The listing builds one solid part. Answer for the finished solid, in the listing's coordinates (mm). Give positions to 0.01 mm unless a question says otherwise; leave off trailing zeros. Write each loop counter-clockwise with the first axis right and the second up, starting at its lowest first coordinate (ties: lowest second). Pieces come first, ordered by that corner, then holes. Notation, with made-up numbers: (-19.75, 13) - (35.25, 13) arc R6 ccw to (35.25, 21) - close; hole circle Ø11 at (39, -26). An arc over 180 degrees is marked (long way). Write each question's results on one line, items separated by ' | '. Start each with the question number.
Q1. Section A-A (z = 0) is taken. Determine the outline of the cut face in (x, y).
Q2. Flat-ended cylindrical pins translate along their axes: pin 1 Ø2 at (y, z) = (2.5, -91) entering from +X; pin 2 Ø2 at (x, y) = (23, 2) entering from +Z. Find the tip coordinate at first contact, or state that the pin passes through.
Q3. Section B-B (y = 0.95) is taken. State how many separate pieces and enclosed holes the cut face has, plus the area to 3 significant figures.
Q4. Find the intervals of material crossed by probe 1 along X at (y, z) = (1, -36.5); probe 2 along Z at (x, y) = (84.5, 2.55); probe 3 along Z at (x, y) = (79.5, 0.35), in increasing order.
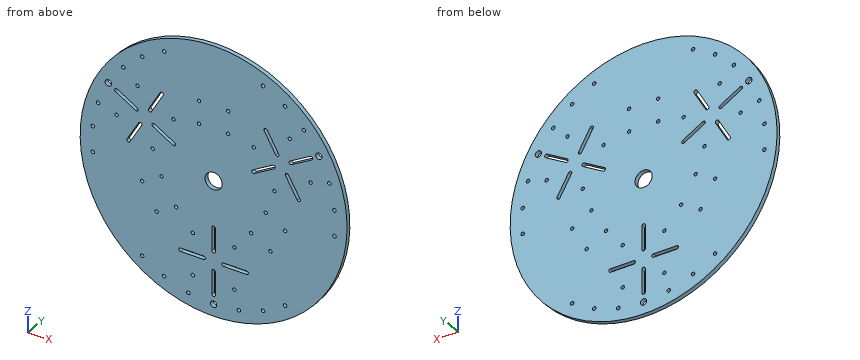
```python
from build123d import *

# Parameters (mm, degrees)
SKETCH1_R           = 125
SKETCH1_R_2         = 8
SKETCH1_R_3         = 2.95
SKETCH1_R_4         = 1.675
SKETCH1_R_5         = 1.6
BOSS_EXTRUDE2_DEPTH = 4


with BuildPart() as part:
    # Sketch1 → Boss-Extrude2 (new body)
    with BuildSketch(Plane(origin=(0, 0, 0), x_dir=(1, 0, 0), z_dir=(0, 1, 0))):
        with Locations(Location((0, 0, 0), (0, 0, 270))):
            Circle(SKETCH1_R)
        with Locations(Location((0, 0, 0), (0, 0, 270))):
            Circle(SKETCH1_R_2, mode=Mode.SUBTRACT)
        with Locations(Location((0, 113.85, 0), (0, 0, 270))):
            Circle(SKETCH1_R_3, mode=Mode.SUBTRACT)
        with Locations(Location((98.596992221, -56.925, 0), (0, 0, 270))):
            Circle(SKETCH1_R_3, mode=Mode.SUBTRACT)
        with Locations(Location((-98.596992221, -56.925, 0), (0, 0, 270))):
            Circle(SKETCH1_R_3, mode=Mode.SUBTRACT)
        with Locations(Location((23.670746, 111.362104344, 0), (0, 0, 270))):
            Circle(SKETCH1_R_4, mode=Mode.SUBTRACT)
        with Locations(Location((46.306966814, 104.007150353, 0), (0, 0, 270))):
            Circle(SKETCH1_R_4, mode=Mode.SUBTRACT)
        with Locations(Location((66.919350973, 92.10658481, 0), (0, 0, 270))):
            Circle(SKETCH1_R_4, mode=Mode.SUBTRACT)
        with Locations(Location((113.226317788, 11.900565543, 0), (0, 0, 270))):
            Circle(SKETCH1_R_4, mode=Mode.SUBTRACT)
        with Locations(Location((113.226317788, -11.900565543, 0), (0, 0, 270))):
            Circle(SKETCH1_R_4, mode=Mode.SUBTRACT)
        with Locations(Location((108.27778438, -35.18158481, 0), (0, 0, 270))):
            Circle(SKETCH1_R_4, mode=Mode.SUBTRACT)
        with Locations(Location((84.607038381, -76.180519534, 0), (0, 0, 270))):
            Circle(SKETCH1_R_4, mode=Mode.SUBTRACT)
        with Locations(Location((66.919350974, -92.10658481, 0), (0, 0, 270))):
            Circle(SKETCH1_R_4, mode=Mode.SUBTRACT)
        with Locations(Location((46.306966814, -104.007150353, 0), (0, 0, 270))):
            Circle(SKETCH1_R_4, mode=Mode.SUBTRACT)
        with Locations(Location((-46.306966814, -104.007150353, 0), (0, 0, 270))):
            Circle(SKETCH1_R_4, mode=Mode.SUBTRACT)
        with Locations(Location((-66.919350973, -92.10658481, 0), (0, 0, 270))):
            Circle(SKETCH1_R_4, mode=Mode.SUBTRACT)
        with Locations(Location((-84.607038381, -76.180519534, 0), (0, 0, 270))):
            Circle(SKETCH1_R_4, mode=Mode.SUBTRACT)
        with Locations(Location((-108.27778438, -35.18158481, 0), (0, 0, 270))):
            Circle(SKETCH1_R_4, mode=Mode.SUBTRACT)
        with Locations(Location((-113.226317788, -11.900565543, 0), (0, 0, 270))):
            Circle(SKETCH1_R_4, mode=Mode.SUBTRACT)
        with Locations(Location((-113.226317788, 11.900565543, 0), (0, 0, 270))):
            Circle(SKETCH1_R_4, mode=Mode.SUBTRACT)
        with Locations(Location((-66.919350973, 92.10658481, 0), (0, 0, 270))):
            Circle(SKETCH1_R_4, mode=Mode.SUBTRACT)
        with Locations(Location((-46.306966814, 104.007150353, 0), (0, 0, 270))):
            Circle(SKETCH1_R_4, mode=Mode.SUBTRACT)
        with Locations(Location((-23.670746, 111.362104344, 0), (0, 0, 270))):
            Circle(SKETCH1_R_4, mode=Mode.SUBTRACT)
        with Locations(Location((-90.831628429, -29.925004626, 0), (0, 0, 270))):
            Circle(SKETCH1_R_5, mode=Mode.SUBTRACT)
        with Locations(Location((-57.056637682, -10.425004626, 0), (0, 0, 270))):
            Circle(SKETCH1_R_5, mode=Mode.SUBTRACT)
        with Locations(Location((-37.556637682, -44.199995374, 0), (0, 0, 270))):
            Circle(SKETCH1_R_5, mode=Mode.SUBTRACT)
        with Locations(Location((-71.331628429, -63.699995374, 0), (0, 0, 270))):
            Circle(SKETCH1_R_5, mode=Mode.SUBTRACT)
        with Locations(Location((19.5, 93.625, 0), (0, 0, 270))):
            Circle(SKETCH1_R_5, mode=Mode.SUBTRACT)
        with Locations(Location((19.5, 54.625, 0), (0, 0, 270))):
            Circle(SKETCH1_R_5, mode=Mode.SUBTRACT)
        with Locations(Location((-19.5, 54.625, 0), (0, 0, 270))):
            Circle(SKETCH1_R_5, mode=Mode.SUBTRACT)
        with Locations(Location((-19.5, 93.625, 0), (0, 0, 270))):
            Circle(SKETCH1_R_5, mode=Mode.SUBTRACT)
        with Locations(Location((71.331628429, -63.699995374, 0), (0, 0, 270))):
            Circle(SKETCH1_R_5, mode=Mode.SUBTRACT)
        with Locations(Location((37.556637682, -44.199995374, 0), (0, 0, 270))):
            Circle(SKETCH1_R_5, mode=Mode.SUBTRACT)
        with Locations(Location((57.056637682, -10.425004626, 0), (0, 0, 270))):
            Circle(SKETCH1_R_5, mode=Mode.SUBTRACT)
        with Locations(Location((90.831628429, -29.925004626, 0), (0, 0, 270))):
            Circle(SKETCH1_R_5, mode=Mode.SUBTRACT)
        with Locations(Location((-13.625, -48.465, 0), (0, 0, 270))):
            Circle(SKETCH1_R_5, mode=Mode.SUBTRACT)
        with Locations(Location((13.625, -48.465, 0), (0, 0, 270))):
            Circle(SKETCH1_R_5, mode=Mode.SUBTRACT)
        with Locations(Location((13.625, -69.465, 0), (0, 0, 270))):
            Circle(SKETCH1_R_5, mode=Mode.SUBTRACT)
        with Locations(Location((-13.625, -69.465, 0), (0, 0, 270))):
            Circle(SKETCH1_R_5, mode=Mode.SUBTRACT)
        with Locations(Location((-35.159421194, 36.032096127, 0), (0, 0, 270))):
            Circle(SKETCH1_R_5, mode=Mode.SUBTRACT)
        with Locations(Location((-48.784421194, 12.432903873, 0), (0, 0, 270))):
            Circle(SKETCH1_R_5, mode=Mode.SUBTRACT)
        with Locations(Location((-66.970954674, 22.932903873, 0), (0, 0, 270))):
            Circle(SKETCH1_R_5, mode=Mode.SUBTRACT)
        with Locations(Location((-53.345954674, 46.532096127, 0), (0, 0, 270))):
            Circle(SKETCH1_R_5, mode=Mode.SUBTRACT)
        with Locations(Location((48.784421194, 12.432903873, 0), (0, 0, 270))):
            Circle(SKETCH1_R_5, mode=Mode.SUBTRACT)
        with Locations(Location((35.159421194, 36.032096127, 0), (0, 0, 270))):
            Circle(SKETCH1_R_5, mode=Mode.SUBTRACT)
        with Locations(Location((53.345954674, 46.532096127, 0), (0, 0, 270))):
            Circle(SKETCH1_R_5, mode=Mode.SUBTRACT)
        with Locations(Location((66.970954674, 22.932903873, 0), (0, 0, 270))):
            Circle(SKETCH1_R_5, mode=Mode.SUBTRACT)
        with BuildLine():
            Line((-71.383217405, -43.060640646), (-90.262571208, -53.960640646))
            ThreePointArc((-90.262571208, -53.960640646), (-92.448211854, -53.375), (-91.862571208, -51.189359354))
            Line((-91.862571208, -51.189359354), (-72.983217405, -40.289359354))
            ThreePointArc((-72.983217405, -40.289359354), (-70.797576759, -40.875), (-71.383217405, -43.060640646))
        make_face(mode=Mode.SUBTRACT)
        with BuildLine():
            Line((-36.525694903, -22.935640646), (-55.405048706, -33.835640646))
            ThreePointArc((-55.405048706, -33.835640646), (-57.590689352, -33.25), (-57.005048706, -31.064359354))
            Line((-57.005048706, -31.064359354), (-38.125694903, -20.164359354))
            ThreePointArc((-38.125694903, -20.164359354), (-35.940054257, -20.75), (-36.525694903, -22.935640646))
        make_face(mode=Mode.SUBTRACT)
        with BuildLine():
            Line((-70.192273702, -29.87341565), (-81.092273702, -10.994061848))
            ThreePointArc((-81.092273702, -10.994061848), (-80.506633056, -8.808421202), (-78.320992409, -9.394061848))
            Line((-78.320992409, -9.394061848), (-67.420992409, -28.27341565))
            ThreePointArc((-67.420992409, -28.27341565), (-68.006633056, -30.459056296), (-70.192273702, -29.87341565))
        make_face(mode=Mode.SUBTRACT)
        with BuildLine():
            Line((-58.195992409, -44.25158435), (-47.295992409, -63.130938152))
            ThreePointArc((-47.295992409, -63.130938152), (-47.881633056, -65.316578798), (-50.067273702, -64.730938152))
            Line((-50.067273702, -64.730938152), (-60.967273702, -45.85158435))
            ThreePointArc((-60.967273702, -45.85158435), (-60.381633056, -43.665943704), (-58.195992409, -44.25158435))
        make_face(mode=Mode.SUBTRACT)
        with BuildLine():
            Line((-1.6, 83.35), (-1.6, 105.15))
            ThreePointArc((-1.6, 105.15), (0, 106.75), (1.6, 105.15))
            Line((1.6, 105.15), (1.6, 83.35))
            ThreePointArc((1.6, 83.35), (0, 81.75), (-1.6, 83.35))
        make_face(mode=Mode.SUBTRACT)
        with BuildLine():
            Line((-1.6, 43.1), (-1.6, 64.9))
            ThreePointArc((-1.6, 64.9), (0, 66.5), (1.6, 64.9))
            Line((1.6, 64.9), (1.6, 43.1))
            ThreePointArc((1.6, 43.1), (0, 41.5), (-1.6, 43.1))
        make_face(mode=Mode.SUBTRACT)
        with BuildLine():
            Line((9.225, 75.725), (31.025, 75.725))
            ThreePointArc((31.025, 75.725), (32.625, 74.125), (31.025, 72.525))
            Line((31.025, 72.525), (9.225, 72.525))
            ThreePointArc((9.225, 72.525), (7.625, 74.125), (9.225, 75.725))
        make_face(mode=Mode.SUBTRACT)
        with BuildLine():
            Line((-9.225, 72.525), (-31.025, 72.525))
            ThreePointArc((-31.025, 72.525), (-32.625, 74.125), (-31.025, 75.725))
            Line((-31.025, 75.725), (-9.225, 75.725))
            ThreePointArc((-9.225, 75.725), (-7.625, 74.125), (-9.225, 72.525))
        make_face(mode=Mode.SUBTRACT)
        with BuildLine():
            Line((72.983217405, -40.289359354), (91.862571208, -51.189359354))
            ThreePointArc((91.862571208, -51.189359354), (92.448211854, -53.375), (90.262571208, -53.960640646))
            Line((90.262571208, -53.960640646), (71.383217405, -43.060640646))
            ThreePointArc((71.383217405, -43.060640646), (70.797576759, -40.875), (72.983217405, -40.289359354))
        make_face(mode=Mode.SUBTRACT)
        with BuildLine():
            Line((38.125694903, -20.164359354), (57.005048706, -31.064359354))
            ThreePointArc((57.005048706, -31.064359354), (57.590689352, -33.25), (55.405048706, -33.835640646))
            Line((55.405048706, -33.835640646), (36.525694903, -22.935640646))
            ThreePointArc((36.525694903, -22.935640646), (35.940054257, -20.75), (38.125694903, -20.164359354))
        make_face(mode=Mode.SUBTRACT)
        with BuildLine():
            Line((60.967273702, -45.85158435), (50.067273702, -64.730938152))
            ThreePointArc((50.067273702, -64.730938152), (47.881633056, -65.316578798), (47.295992409, -63.130938152))
            Line((47.295992409, -63.130938152), (58.195992409, -44.25158435))
            ThreePointArc((58.195992409, -44.25158435), (60.381633056, -43.665943704), (60.967273702, -45.85158435))
        make_face(mode=Mode.SUBTRACT)
        with BuildLine():
            Line((67.420992409, -28.27341565), (78.320992409, -9.394061848))
            ThreePointArc((78.320992409, -9.394061848), (80.506633056, -8.808421202), (81.092273702, -10.994061848))
            Line((81.092273702, -10.994061848), (70.192273702, -29.87341565))
            ThreePointArc((70.192273702, -29.87341565), (68.006633056, -30.459056296), (67.420992409, -28.27341565))
        make_face(mode=Mode.SUBTRACT)
    extrude(amount=BOSS_EXTRUDE2_DEPTH)


solid = part.part
```
Answers below:
1) outline: (-125, 0) - (-8, 0) - (-8, 4) - (-125, 4) - close; (8, 0) - (125, 0) - (125, 4) - (8, 4) - close
2) pin 1: stops at x = 86.75 | pin 2: stops at z = 123.05
3) separate pieces: 1 | enclosed holes: 58 | area: 47,500 mm2
4) probe 1: x = -119.55 to -36.69, -33.63 to 33.63, 36.69 to 119.55 | probe 2: z = -92.11 to 46.94, 50.63 to 74.51, 77.85 to 92.11 | probe 3: z = -96.46 to 8.61, 13.75 to 44.05, 47.75 to 96.46
